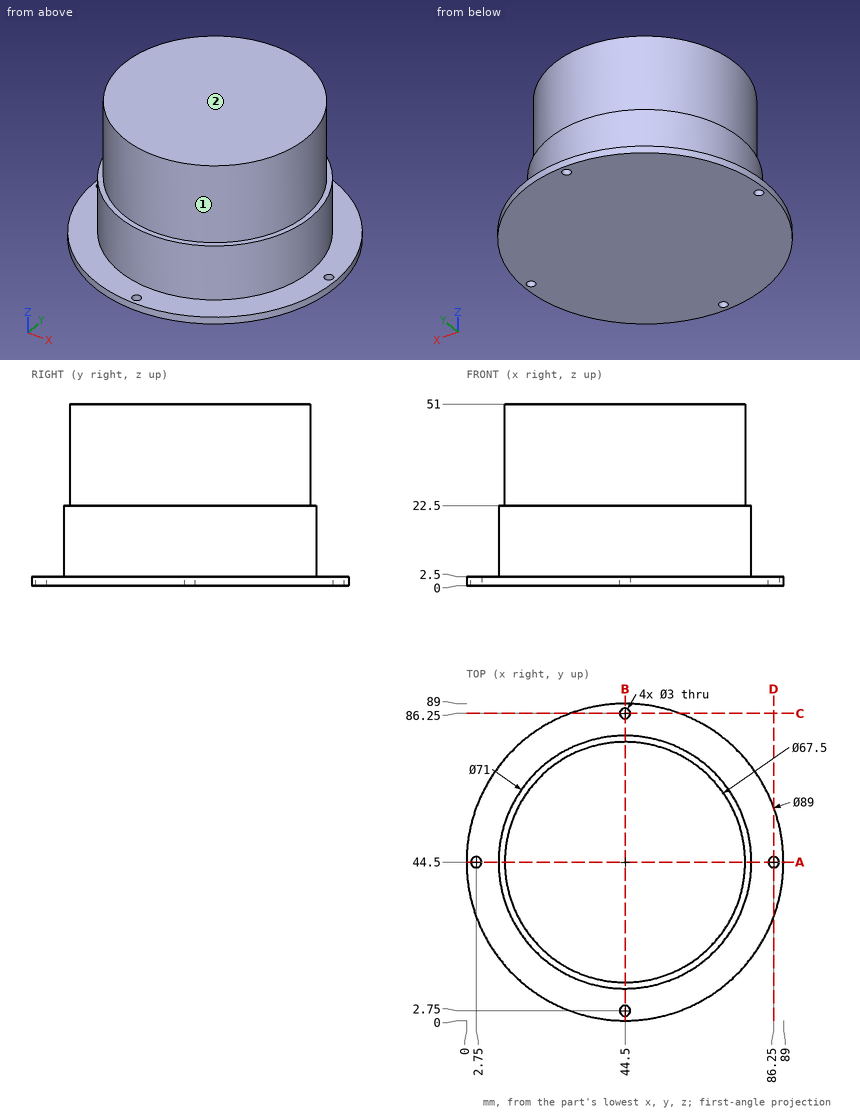
Here's the drawing with two shaded views (mm, measured from the low corner). I have some questions. A direction names the side the tool comes from. Coordinates: 2 decimals unless noted, no trailing zeros. Write each loop counter-clockwise with the first axis right and the second up, starting at its lowest first coordinate (ties: lowest second). Pieces come first, ordered by that corner, then holes. Notation, with made-up numbers: (36.5, 68) -> (56.5, 68) arc R22 cw to (56.5, 100) -> close; hole circle Ø4 at (40, -3). An arc over 180 degrees is marked (long way). Write item = value, one per line. Start each with the question number.
(1) I need wall thicknesses on line 1 (Y direction, x = 44, z = 1); line 2 (Z direction, x = 67.5, y = 80.5); line 3 (X direction, y = 28.5, z = 23). Which ranges of each line are inside material? Lowest first, please. Write a range as [from, to].
(2) Which directions (+Z, -Z, +X, -X, +Y, -Y) give clear straight access to the entire face, cutting with the end or side of a thin tool? Please do the marked faces 1 and 2.
(3) I want a section at C-C (y = 86.25). Please give me the cut outline in (x, z), plus the area to 3 significant figures.
(4) Will these pins go through, and if not, where does the flat tip stop? pin 1 (1 mm diameter, centred on x = 28, z = 29.5, fed in from -Y); pin 2 (1 mm diameter, centred on y = 40.5, z = 45.5, fed in from -X); pin 3 (8 mm diameter, centred on x = 35.5, z = 8, fed in from -Y).
(5) I want a section at A-A (y = 44.5). Please give me the cut outline in (x, z), plus the area to 3 significant figures.
Result set:
q1.line_1 = [0, 1.34], [4.16, 84.84], [87.66, 89]
q1.line_2 = [0, 2.5]
q1.line_3 = [14.78, 74.22]
q2.face_1 = +Z
q2.face_2 = +Z, +X, -X, +Y, -Y
q3.outline = (29.1, 0) -> (43, 0) -> (43, 2.5) -> (29.1, 2.5) -> close; (46, 0) -> (59.9, 0) -> (59.9, 2.5) -> (46, 2.5) -> close
q3.area = 69.5 mm2
q4.pin_1 = 14.78
q4.pin_2 = 10.93
q4.pin_3 = 9.35
q5.outline = (0, 0) -> (1.25, 0) -> (1.25, 2.5) -> (0, 2.5) -> close; (4.25, 0) -> (84.75, 0) -> (84.75, 2.5) -> (80, 2.5) -> (80, 22.5) -> (78.25, 22.5) -> (78.25, 51) -> (10.75, 51) -> (10.75, 22.5) -> (9, 22.5) -> (9, 2.5) -> (4.25, 2.5) -> close; (87.75, 0) -> (89, 0) -> (89, 2.5) -> (87.75, 2.5) -> close
q5.area = 3,550 mm2
